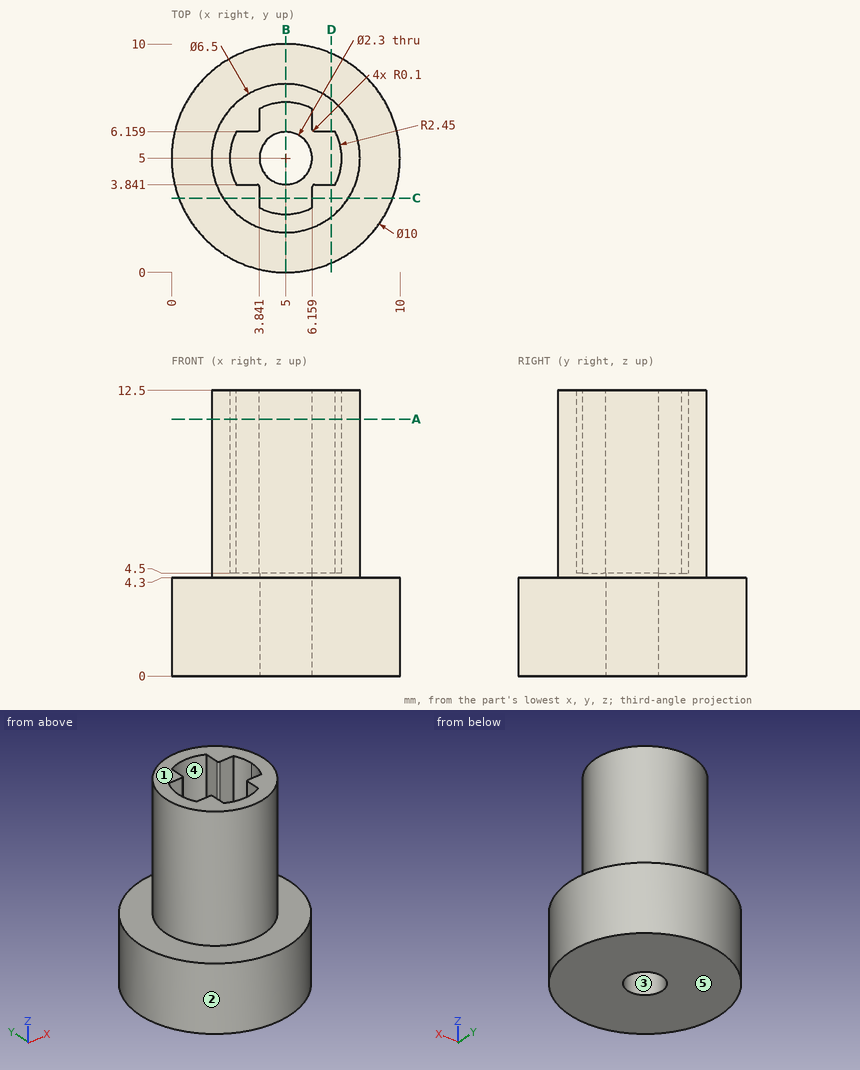
Geometry: see drawing. Coordinates: mm, zero at the bounding-box minimum. A direction names the side the tool comes from. Give positions to 0.01 mm unless a question says otherwise; leave off trailing zeros. Order: outer loops, then holes, each group sorted by start corner. A loop starts at its lowest first (then second) coordinate and runs counter-clockwise, first axis right, second up.
Q1. Section C-C on y = 3.25. Output: boundary loops of the cut face in (x, z).
Checked values:
outline: (0.32, 0) - (9.68, 0) - (9.68, 4.3) - (7.74, 4.3) - (7.74, 12.5) - (6.16, 12.5) - (6.16, 4.5) - (3.84, 4.5) - (3.84, 12.5) - (2.26, 12.5) - (2.26, 4.3) - (0.32, 4.3) - close
Q2. Draft query along Y for the marked faces 1, 2 and 3. Return one class per face: +Y half, -Y half, draft (parallel to the pull), parting line (faces both ways), or undercut.
Checked values:
face 1: draft
face 2: parting line
face 3: undercut
Q3. Set-up query: the marked faces 4 and 5. Return all of +Z, -Z, +X, -X, +Y, -Y with unobstructed straight access to the full face (end or side cutting, diameter ignored); none if empty.
Checked values:
face 4: +Z
face 5: -Z, +X, -X, +Y, -Y
Q4. Section D-D on x = 7. Output: boundary loops of the cut face in (y, z).
Checked values:
outline: (0.42, 0) - (9.58, 0) - (9.58, 4.3) - (7.56, 4.3) - (7.56, 12.5) - (6.16, 12.5) - (6.16, 4.5) - (3.84, 4.5) - (3.84, 12.5) - (2.44, 12.5) - (2.44, 4.3) - (0.42, 4.3) - close
Q5. Contact query for flat-ended pins moving along their axis: pin 1 Ø0.7 at (y, z) = (6.5, 8.5) entering from +X; pin 2 Ø1.8 at (x, y) = (5, 5) entering from +Z; pin 3 Ø4 at (y, z) = (4, 9) entering from -X; pin 4 Ø0.5 at (x, z) = (6.5, 9.5) entering from +Y. Output: stop coordinate, or through.
Checked values:
pin 1: stops at x = 8.04
pin 2: passes through
pin 3: stops at x = 1.75
pin 4: stops at y = 8
Q6. Section B-B on x = 5. Output: boundary loops of the cut face in (y, z).
Checked values:
outline: (0, 0) - (3.85, 0) - (3.85, 4.5) - (2.55, 4.5) - (2.55, 12.5) - (1.75, 12.5) - (1.75, 4.3) - (0, 4.3) - close; (6.15, 0) - (10, 0) - (10, 4.3) - (8.25, 4.3) - (8.25, 12.5) - (7.45, 12.5) - (7.45, 4.5) - (6.15, 4.5) - close
Q7. Section A-A on z = 11.25. Output: boundary loops of the cut face in (x, y), and give its area (3 significant figures).
Checked values:
outline: circle Ø6.5 at (5, 5); hole (2.84, 3.84) - (3.74, 3.84) arc R0.1 cw to (3.84, 3.74) - (3.84, 2.84) arc R2.45 ccw to (6.16, 2.84) - (6.16, 3.74) arc R0.1 cw to (6.26, 3.84) - (7.16, 3.84) arc R2.45 ccw to (7.16, 6.16) - (6.26, 6.16) arc R0.1 cw to (6.16, 6.26) - (6.16, 7.16) arc R2.45 ccw to (3.84, 7.16) - (3.84, 6.26) arc R0.1 cw to (3.74, 6.16) - (2.84, 6.16) arc R2.45 ccw to start
area: 16.7 mm2
Q8. Ray query, probe 1 along Y at (x, z) = (5, 2.35); probe 2 along Z at (x, y) = (4.25, 9.75); probe 3 along Z at (x, y) = (4.25, 7). Return the intervals inside material, ascending.
Checked values:
probe 1: y = 0 to 3.85, 6.15 to 10
probe 2: z = 0 to 4.3
probe 3: z = 0 to 4.5
